Could you check a few things on this model? Use its own coordinates, in mm. A direction names the side the tool comes from. Give positions to 0.01 mm unless a question says otherwise; leave off trailing zeros. Write each loop counter-clockwise with the first axis right and the second up, starting at its lowest first coordinate (ties: lowest second). Pieces come first, ordered by that corner, then holes. Notation, with made-up numbers: (77, 50.5) -> (98, 50.5) arc R16 cw to (98, 73.5) -> close; hole circle Ø8 at (3, 27). An arc over 180 degrees is marked (long way). One line per question, with ' | ' between items.
from build123d import *

# Parameters (mm, degrees)
PAD003_DEPTH       = 5
PAD004_DEPTH       = 0.5
HOLE_D             = 3.4
HOLE_DEPTH         = 25
HOLE_CBORE_D       = 7
HOLE_CBORE_DEPTH   = 3.4
POLARPATTERN_COUNT = 6


with BuildPart() as part:
    # Sketch005 → Pad003 (new body)
    with BuildSketch(Plane.XY):
        Polygon((73.30127, 42.320508), (0, 84.641016), (-73.30127, 42.320508), (-73.30127, -42.320508), (0, -84.641016), (73.30127, -42.320508), align=None)
        Polygon((58.30127, 33.660254), (0, 67.320508), (-58.30127, 33.660254), (-58.30127, -33.660254), (0, -67.320508), (58.30127, -33.660254), align=None, mode=Mode.SUBTRACT)
    extrude(amount=PAD003_DEPTH)

    # Sketch006 (on Face14 of Pad003) → Pad004 (join)
    with BuildSketch(Plane.XY.offset(5)):
        Polygon((-73.30127, 42.320508), (-73.30127, -42.320508), (0, -84.641016), (73.30127, -42.320508), (73.30127, 42.320508), (0, 84.641016), align=None)
    extrude(amount=PAD004_DEPTH)

    # Hole
    with Locations(Plane.XY.offset(5.5)):
        with Locations((-34.150635, 59.150635)):
            hole = CounterBoreHole(HOLE_D / 2, HOLE_CBORE_D / 2, HOLE_CBORE_DEPTH, depth=HOLE_DEPTH)

    # PolarPattern: Hole ×6 about axis
    polarpattern_axis = Axis((0, 0, 0), (0, 0, 1))
    for i in range(1, POLARPATTERN_COUNT):
        add(hole.rotate(polarpattern_axis, i * 360 / POLARPATTERN_COUNT), mode=Mode.SUBTRACT)


with BuildPart() as part_1:
    # Body002 placement: moved
    add(part.part.moved(Location((0, 0, 17))))


solid = part_1.part
Q1. Imagine slicing it at D-D on x = -61.5. Please give me the cut outline in (y, z).
Answer below:
outline: (-49.13, 17) -> (49.13, 17) -> (49.13, 22.5) -> (-49.13, 22.5) -> close
Q2. If we mould it in two halves opening along X, with no side actions, what happens to faces 1 (the cylindrical face through (-35.72, 58.5, 18.04)), 2 (the flat face through (-1, 1, 22.5)), 3 (the flat face through (-36.1, 63.8, 19.7))? For each: +X half, -X half, draft (parallel to the pull), parting line (faces both ways), or undercut.
Answer below:
face 1: undercut | face 2: draft | face 3: -X half
Q3. On a 3-axis mill with a long thin cutter (end or side, diameter ignored), from which of +Z, -Z, +X, -X, +Y, -Y can I reach the whole of each face in a straight line? I mean faces 4 (the flat face through (-37.164, -63.185, 19.712)), 5 (the flat face through (36, -58, 19.1)), 6 (the flat face through (30, 50, 19)). Say none if no direction works.
Answer below:
face 4: +Z, -Z, -X, -Y | face 5: +Z | face 6: -Z
Q4. If I drill on line 1 along X through (y, z) = (14, 21.55); line 2 along Z through (x, y) = (23.5, 11.5); line 3 along X through (y, z) = (58, 20.5), over which ranges is the centre line in solid material (lowest first)?
Answer below:
line 1: x = -73.3 to -58.3, 58.3 to 73.3 | line 2: z = 22 to 22.5 | line 3: x = -46.14 to -37.46, -30.85 to -16.14, 16.14 to 30.85, 37.46 to 46.14
Q5. Imagine slicing it at B-B on z = 20.9. Please give me the cut outline in (x, y).
Answer below:
outline: (-73.3, -42.32) -> (0, -84.64) -> (73.3, -42.32) -> (73.3, 42.32) -> (0, 84.64) -> (-73.3, 42.32) -> close; hole circle Ø7 at (-68.3, 0); hole (-58.3, -33.66) -> (0, -67.32) -> (58.3, -33.66) -> (58.3, 33.66) -> (0, 67.32) -> (-58.3, 33.66) -> close; hole circle Ø7 at (-34.15, -59.15); hole circle Ø7 at (-34.15, 59.15); hole circle Ø7 at (34.15, -59.15); hole circle Ø7 at (34.15, 59.15); hole circle Ø7 at (68.3, 0)
Q6. Imagine slicing it at C-C on x = 25. Please give me the cut outline in (y, z).
Answer below:
outline: (-70.21, 17) -> (-52.89, 17) -> (-52.89, 22) -> (52.89, 22) -> (52.89, 17) -> (70.21, 17) -> (70.21, 22.5) -> (-70.21, 22.5) -> close
Q7. Will these pins go through, and if not, where does the flat tip stop? pin 1 (4 mm diameter, centred on x = -34.15, y = -59.15, fed in from +Z); pin 2 (3 mm diameter, centred on y = -48, z = 22, fed in from -X); pin 3 (6.5 mm diameter, centred on x = 68.3, y = 0, fed in from -Z); pin 4 (3 mm diameter, centred on x = 21.5, y = 5.5, fed in from -Z).
Answer below:
pin 1: stops at z = 19.1 | pin 2: stops at x = -66.06 | pin 3: stops at z = 17 | pin 4: stops at z = 22
Q8. Imagine slicing it at A-A on y = 15. Please give me the cut outline in (x, z), and give its area (3 significant figures).
Answer below:
outline: (-73.3, 17) -> (-58.3, 17) -> (-58.3, 22) -> (58.3, 22) -> (58.3, 17) -> (73.3, 17) -> (73.3, 22.5) -> (-73.3, 22.5) -> close | area: 223 mm^2
